Read the model definition and answer for the solid it produces. Units are mm, in the model's axes. A direction names the side the tool comes from. Round coordinates to 2 decimals unless told otherwise and drop trailing zeros. Loops run counter-clockwise (first coordinate to the right, second up) from the corner with the lowest first, then second, coordinate; pieces in that order, holes last. Notation, with made-up numbers: M 77,-1.5 L 93,-1.5 A28 cw 93,29.5 Z; hole C 46,39 d9. An arc over 180 degrees is marked long. Write each question's results on one line, items separated by ' | '.
Autodesk Inventor part; units mm, degrees
ref_plane "YZ Plane" through (0, 0, 0) normal (1, 0, 0) x (0, 1, 0)
ref_plane "XZ Plane" through (0, 0, 0) normal (0, 1, 0) x (-1, 0, 0)
ref_plane "XY Plane" through (0, 0, 0) normal (0, 0, 1) x (1, 0, 0)
sketch "Sketch1" plane through (0, 0, 0) normal (0, 0, 1) x (1, 0, 0)
  circle A0 centre (0, 0) radius 11
  circle A1 centre (0, 0) radius 2
  dimension "d0" = 22
  dimension "d1" = 4
extrude "Extrusion1" add sketch "Sketch1" along normal blind 6.5
sketch "Sketch2" plane through (0, 0, 6.5) normal (0, 0, 1) x (1, 0, 0)
  circle A0 centre (0, 0) radius 9
  circle A1 centre (0, 0) radius 2
  dimension "d4" = 18
extrude "Extrusion2" add sketch "Sketch2" along normal blind 5.5
sketch "Sketch3" plane through (0, 0, 12) normal (0, 0, 1) x (1, 0, 0)
  circle A0 centre (-5.4177, 3.0147) radius 1.5
  circle A1 centre (0.098, -6.1992) radius 1.5
  circle A2 centre (5.3197, 3.1845) radius 1.5
  circle A3 centre (0, 0) radius 6.2 construction
  dimension "d21" = 12.4
  dimension "d7" = 3
  dimension "d10" = 360
extrude "Extrusion3" cut sketch "Sketch3" against normal through all
sketch "Sketch4" plane through (0, 0, 0) normal (0, 1, 0) x (-1, 0, 0)
  circle A0 centre (0, 9.25) radius 2
  circle A1 centre (0, 3.25) radius 2
  line L0 (0, 0) -> (0, 21.1328) construction
  dimension "d15" = 4
  dimension "d16" = 4
  dimension "d17" = 3.25
  dimension "d18" = 9.25
extrude "Extrusion4" cut sketch "Sketch4" along normal through all
thread "Thread1"
thread "Thread2"
thread "Thread3"
thread "Thread4"
thread "Thread5"
properties part number "WheelAdapter-4mm" material "Aluminum 6061"
Item 1: Flat-ended cylindrical pins translate along their axes: pin 1 (3.5 mm diameter, centred on x = 0, z = 3.25, fed in from +Y); pin 2 (3 mm diameter, centred on x = -2, z = 8.5, fed in from -Y); pin 3 (1 mm diameter, centred on y = -1, z = 8.5, fed in from +X); pin 4 (2.5 mm diameter, centred on x = -5.42, y = 3.01, fed in from -Z). Find the tip coordinate at first contact, or state that the pin passes through.
Outcome:
pin 1: stops at y = -0.97 | pin 2: stops at y = -8.99 | pin 3: stops at x = 8.99 | pin 4: passes through
Item 2: The mould has two halves that part along Y. Classify faces 4 (the face through (-2.38, 10.74, 3.2)), 5 (the face through (0.79, -7.53, 6.08)), 6 (the face through (1.474, 6.646, 1.898)): pulls with the +Y half, pulls with the -Y half, needs draft (parallel to the pull), parting line crosses it, or undercut.
Outcome:
face 4: parting line crosses it | face 5: undercut | face 6: needs draft
Item 3: The part is cut by section B-B (x = -5). Determine the outline of the cut face in (y, z), plus the area to 3 significant figures.
Outcome:
outline: M -9.8,0 L 1.57,0 L 1.57,12 L -7.48,12 L -7.48,6.5 L -9.8,6.5 Z; M 4.46,0 L 9.8,0 L 9.8,6.5 L 7.48,6.5 L 7.48,12 L 4.46,12 Z | area: 175 mm2
Item 4: The part is cut by section A-A (y = -6.5). Determine the outline of the cut face in (x, z).
Outcome:
outline: M -8.87,0 L -1.37,0 L -1.37,12 L -6.22,12 L -6.22,6.5 L -8.87,6.5 Z; M 1.57,0 L 8.87,0 L 8.87,6.5 L 6.22,6.5 L 6.22,12 L 1.57,12 Z
Item 5: The part is cut by section D-D (x = 0). Determine the outline of the cut face in (y, z), plus the area to 3 significant figures.
Outcome:
outline: M -11,0 L -7.7,0 L -7.7,12 L -9,12 L -9,6.5 L -11,6.5 Z; M -4.7,0 L -2,0 L -2,12 L -4.7,12 Z; M 2,0 L 11,0 L 11,1.25 L 2,1.25 Z; M 2,5.25 L 11,5.25 L 11,6.5 L 9,6.5 L 9,7.25 L 2,7.25 Z; M 2,11.25 L 9,11.25 L 9,12 L 2,12 Z | area: 94.1 mm2
Item 6: For faces 1 (the face through (-1.172, -8.923, 9.212)), 2 (the face through (0, -2, 6)), 3 (the face through (2, 5.4, 9.2)), determine the directions among +Z, -Z, +X, -X, +Y, -Y from which every point of the face is accessible in a straight line to the end or side of a thin tool.
Outcome:
face 1: +Z | face 2: +Z, -Z | face 3: +Y
Item 7: Straight lines are drawn through the part: line 1 (X direction, y = 2.5, z = 9.25); line 2 (Y direction, x = -1, z = 1); line 3 (Z direction, x = 1, y = 3). For each, find the intervals that lie inside material, in ascending order.
Outcome:
line 1: x = -8.65 to -6.83, -4.01 to -2, 2 to 3.98, 6.65 to 8.65 | line 2: y = -10.95 to -7.22, -5.18 to -1.73, 1.73 to 10.95 | line 3: z = 0 to 1.52, 4.98 to 7.52, 10.98 to 12
Item 8: The part is cut by section C-C (z = 5.75). Determine the outline of the cut face in (x, y), plus the area to 3 significant figures.
Outcome:
outline: C 0,0 d22; hole C -5.42,3.01 d3; hole C 0,0 d4; hole C 0.1,-6.2 d3; hole C 5.32,3.18 d3 | area: 346 mm2
